```python
from build123d import *

# Parameters (mm, degrees)
SKETCH_R        = 20
SKETCH_R_2      = 8
PAD_DEPTH       = 8
SKETCH001_R     = 2.4
SKETCH001_R_2   = 2.3
SKETCH001_R_3   = 1.630743
SKETCH001_R_4   = 1.492514
SKETCH001_R_5   = 2.2
SKETCH001_R_6   = 1.821083
POCKET_DEPTH    = 6
SKETCH002_R     = 19.1322603564
SKETCH002_R_2   = 8.424409
PAD001_DEPTH    = 1.5
SKETCH003_W     = 43.022533
SKETCH003_H     = 0.75
POCKET001_DEPTH = 7.95
SKETCH007_W     = 7.6375744751
SKETCH007_H     = 10.86069433
SKETCH007_W_2   = 8.2446434751
SKETCH007_H_2   = 12.05515533
SKETCH007_W_3   = 8.5299164751
SKETCH007_H_3   = 10.94123533
SKETCH007_W_4   = 11.8328734751
SKETCH007_H_4   = 10.66832833
POCKET002_DEPTH = 8.001
SKETCH008_R     = 1.4
POCKET003_DEPTH = 27.65392667


with BuildPart() as part:
    # Sketch → Pad (new body)
    with BuildSketch(Plane.XY):
        Circle(SKETCH_R)
        Circle(SKETCH_R_2, mode=Mode.SUBTRACT)
    extrude(amount=PAD_DEPTH)

    # Sketch001 (on Face4 of Pad) → Pocket (cut)
    with BuildSketch(Plane.XY.offset(8)):
        with Locations((0, 14)):
            Circle(SKETCH001_R)
        with Locations((-7.5, 12.9903810568)):
            Circle(SKETCH001_R_2)
        with Locations((-17.083683, 37.568653)):
            Circle(SKETCH001_R_3)
        with Locations((9.573956, 39.229813)):
            Circle(SKETCH001_R_4)
        with Locations((9.1772229816, 13.1064327086)):
            Circle(SKETCH001_R_5)
        with Locations((30.140682, 32.901588)):
            Circle(SKETCH001_R_6)
    pocket = extrude(amount=-POCKET_DEPTH, mode=Mode.SUBTRACT)

    # Mirrored: Pocket across Sketch001 H_Axis
    add(pocket.mirror(Plane(origin=(0, 0, 8), x_dir=(0, 0, 1), z_dir=(0, 1, 0))), mode=Mode.SUBTRACT)

    # Sketch002 → Pad001 (join)
    with BuildSketch(Plane.XY.offset(8)):
        Circle(SKETCH002_R)
        Circle(SKETCH002_R_2, mode=Mode.SUBTRACT)
    extrude(amount=-PAD001_DEPTH)

    # Sketch003 → Pocket001 (cut)
    with BuildSketch(Plane.XY.offset(8)):
        with Locations((-0.7364995, 0)):
            Rectangle(SKETCH003_W, SKETCH003_H)
    extrude(amount=-POCKET001_DEPTH, mode=Mode.SUBTRACT)

    # Sketch007 → Pocket002 (cut, through all)
    with BuildSketch(Plane.XY.offset(8)):
        with Locations((-16.7398847624, -13.083273835)):
            Rectangle(SKETCH007_W, SKETCH007_H)
        with Locations((-17.0434192624, 13.680504335)):
            Rectangle(SKETCH007_W_2, SKETCH007_H_2)
        with Locations((17.1860557624, 13.123544335)):
            Rectangle(SKETCH007_W_3, SKETCH007_H_3)
        with Locations((18.8375342624, -12.987090835)):
            Rectangle(SKETCH007_W_4, SKETCH007_H_4)
    extrude(amount=-POCKET002_DEPTH, mode=Mode.SUBTRACT)

    # Sketch008 (on Face19 of Pocket002) → Pocket003 (cut, through all)
    with BuildSketch(Plane(origin=(0, 7.65292667, 0), x_dir=(-1, 0, 0), z_dir=(0, 1, 0))):
        with Locations((-15.963433, 4)):
            Circle(SKETCH008_R)
        with Locations((15.963433, 4)):
            Circle(SKETCH008_R)
    extrude(amount=-POCKET003_DEPTH, mode=Mode.SUBTRACT)


solid = part.part
```
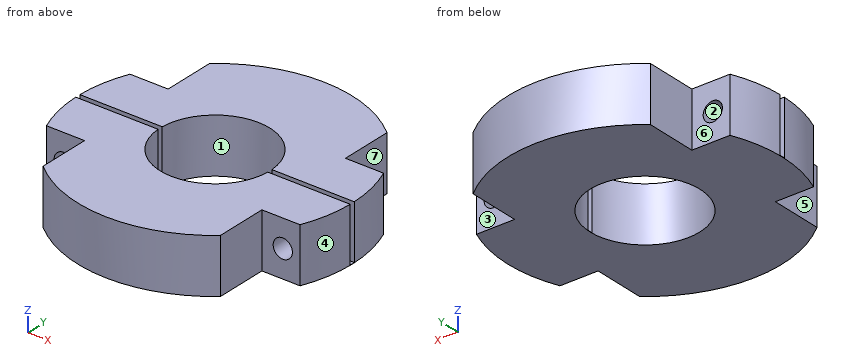
Can you work these out from the model? Positions are in its coordinate system, mm. Face numbers are marked on the shaded views. A direction names the side the tool comes from. Give positions to 0.01 mm unless a question says otherwise; leave off trailing zeros. Loops run counter-clockwise (first coordinate to the right, second up) from the corner with the lowest first, then second, coordinate; pieces in that order, holes last. Notation, with made-up numbers: M 57,83.5 L 66,83.5 A24 cw 66,98.5 Z; hole C 52.25,-26.75 d5. An arc over 180 degrees is marked long. Use CSV: the item, a comma, the result in double quotes. Start each with the question number.
1. If we mould it in two halves opening along X, with no side actions, what happens to the marked faces 1, 2, 3 and 4? For each: released by +X, released by -X, zero draft, split by the parting line, or undercut.
2. If I drill on L1, parallel to Y at x = 18, z = 5.5 (3 decimals); L2, parallel to X at y = 4, z = 5; L3, parallel to X at y = -14, z = 2.75, over which ranges is the centre line in solid material (lowest first)?
3. Imagine slicing it at B-B, the plane y = 4. Write out the boundary of the cut face in (x, z).
4. Imagine slicing it at A-A, the plane x = 0. Write out the boundary of the cut face in (y, z).
5. Imagine slicing it at C-C, the plane z = 0.75. Write out the boundary of the cut face in (x, y) (3 decimals).
6. Imagine slicing it at D-D, the plane x = 4.5. Write out the boundary of the cut face in (y, z).
7. For P1, Ø2.5, axis at x = 12, z = 3.5, coming from the +Y side; P2, Ø4.5, axis at x = 15.96, z = 4, coming from the +Y side; P3, Ø2, axis at y = -12, z = 5.5, coming from the +X side; P4, Ø1.7, axis at x = -15.96, z = 4, coming from the +Y side, each with a flat end and sliding along its axis, tell me the tip position at first contact or that it passes through.
8. On a 3-axis mill with a long thin cutter (end or side, diameter ignored), from which of +Z, -Z, +X, -X, +Y, -Y can I reach the whole of each face in a straight line? I mean the marked faces 5, 6 and 7. Say none if no direction works.
Response values:
1,face 1,"undercut"
1,face 2,"undercut"
1,face 3,"zero draft"
1,face 4,"released by +X"
2,L1,"-7.653 to -0.375, 0.375 to 7.653"
2,L2,"-19.6 to -16.94, -14.98 to -6.93, 6.93 to 14.98, 16.94 to 19.6"
2,L3,"-12.92 to -9.57, -5.43 to -2.4, 2.4 to 7.17, 11.19 to 12.92"
3,outline,"M -19.6,0 L -6.93,0 L -6.93,8 L -19.6,8 Z; M 6.93,0 L 19.6,0 L 19.6,8 L 6.93,8 Z; hole C -15.96,4 d2.8; hole C 15.96,4 d2.8"
4,outline,"M -20,0 L -8,0 L -8,8 L -20,8 Z; M 8,0 L 20,0 L 20,8 L 8,8 Z; hole M -16.4,2 L -11.6,2 L -11.6,6.5 L -16.4,6.5 Z; hole M 11.6,2 L 16.4,2 L 16.4,6.5 L 11.6,6.5 Z"
5,outline,"M -19.996,-0.375 A20 ccw -18.478,-7.653 L -12.921,-7.653 L -12.921,-15.266 A20 ccw 12.921,-15.266 L 12.921,-7.653 L 18.478,-7.653 A20 ccw 19.996,-0.375 L 7.991,-0.375 A8 cw -7.991,-0.375 Z; M -19.996,0.375 L -7.991,0.375 A8 cw 7.991,0.375 L 19.996,0.375 A20 ccw 18.478,7.653 L 12.921,7.653 L 12.921,15.266 A20 ccw -12.921,15.266 L -12.921,7.653 L -18.478,7.653 A20 ccw Z"
6,outline,"M -19.49,0 L -6.61,0 L -6.61,8 L -19.49,8 Z; M 6.61,0 L 19.49,0 L 19.49,8 L 6.61,8 Z"
7,P1,"y = 16.87"
7,P2,"y = 7.65"
7,P3,"x = 12.92"
7,P4,"through"
8,face 5,"+Z, -Z, -X, -Y"
8,face 6,"+Z, -Z, -X, +Y"
8,face 7,"+Z, -Z, +X, +Y"
